from build123d import *

# Parameters (mm, degrees)
F0_R      = 42.199156
F1_DEPTH  = 50.8
F2_R      = 26.140573
F3_DEPTH  = 25.4
F4_R      = 17.712335
F5_DEPTH  = 25.4
F6_R      = 23.120753
F1_FACE_R = 42.199156
F7_DEPTH  = 50.8
F8_R      = 26.373647
F9_DEPTH  = 76.2
F10_R     = 19.05
F11_DEPTH = 254
F12_R     = 5.08


with BuildPart() as f1:
    # F0 (on Front) → F1 (new body)
    with BuildSketch(Plane.XZ):
        Circle(F0_R)
    extrude(amount=F1_DEPTH)

    # F2 (on Front) → F3 (join)
    with BuildSketch(Plane.XZ):
        Circle(F2_R)
    extrude(amount=F3_DEPTH)

    # F4 (on Front) → F5 (join)
    with BuildSketch(Plane.XZ):
        Circle(F4_R)
    extrude(amount=F5_DEPTH)

    # F6 (on Front) + F1_face (on face) → F7 (join)
    with BuildSketch(Plane.XZ):
        Circle(F6_R)
    with BuildSketch(Plane.XZ.offset(50.8)):
        Circle(F1_FACE_R)
    extrude(amount=F7_DEPTH)

    # F8 (on face) → F9 (join)
    with BuildSketch(Plane.XZ.offset(101.6)):
        Circle(F8_R)
    extrude(amount=F9_DEPTH)

    # F10 (on face) → F11 (cut)
    with BuildSketch(Plane.XZ.offset(177.8)):
        Circle(F10_R)
    extrude(amount=-F11_DEPTH, mode=Mode.SUBTRACT)

    # F12
    f12_edges = [f1.edges().sort_by_distance(p)[0] for p in [
        (-26.373647, -177.8, 0),
    ]]
    fillet(f12_edges, radius=F12_R)


solid = f1.part
Work out the finished part from the listing and answer in its coordinate system (mm). A direction names the side the tool comes from. Round coordinates to 2 decimals unless told otherwise and drop trailing zeros. Order: outer loops, then holes, each group sorted by start corner. A loop starts at its lowest first (then second) coordinate and runs counter-clockwise, first axis right, second up. Notation, with made-up numbers: M 24,51.25 L 41,51.25 A19 cw 41,74.25 Z; hole C 13.5,14 d4. An arc over 180 degrees is marked long. Put each result on its own line as item: value. Start each with the question number.
Q1. Straight lines are drawn through the part: L1, parallel to Z at x = 0, y = -87; L2, parallel to Z at x = 0, y = -141; L3, parallel to Y at x = 15.5, z = 34. For each, find the intervals that lie inside material, in ascending order. Write a range as [from, to].
Q2. Section A-A, the plane x = 0 is taken. Write down the section's boundary in (y, z).
Q3. Section C-C, the plane y = -38 is taken. Write down the section's boundary in (x, z).
Q4. Flat-ended cylindrical pins translate along their axes: pin 1 (12 mm diameter, centred on x = -25, y = -21, fed in from +Z); pin 2 (5 mm diameter, centred on x = 1, y = -142.5, fed in from +Z); pin 3 (4 mm diameter, centred on x = 11.5, y = -60, fed in from -Z); pin 4 (12 mm diameter, centred on x = 22, z = 15.5, fed in from -Y). Find the tip coordinate at first contact, or state that the pin passes through.
Q5. Section B-B, the plane z = 0 is taken. Write down the section's boundary in (x, y).
Q6. Section D-D, the plane x = 29 is taken. Write down the section's boundary in (y, z), and give its area (3 significant figures).
Q7. For a pull along X with two mould halves and no side action, classify faces 1 (the cylindrical face through (-5.717, -136.662, -25.746)), 2 (the cylindrical face through (-15.12, -90.14, -11.59)), 3 (the flat face through (18, 0, -9)) as pulls with the +X half, pulls with the -X half, needs draft (parallel to the pull), parting line crosses it, or undercut.
Q8. A tool of negligible diameter and unlimited length cuts with its end or side. For faces 4 (the flat face through (-16, -177.8, -11)), 5 (the flat face through (-19.3, -101.6, -18.2)), from which of +Z, -Z, +X, -X, +Y, -Y can it reach the whole face along a straight path? Write none if from no direction.
Findings below:
1. L1: z = [-42.2, -19.05], [19.05, 42.2]
1. L2: z = [-26.37, -19.05], [19.05, 26.37]
1. L3: y = [-101.6, 0]
2. outline: M -177.8,-21.29 A5.08 ccw -172.72,-26.37 L -101.6,-26.37 L -101.6,-42.2 L 0,-42.2 L 0,-19.05 L -177.8,-19.05 Z; M -177.8,19.05 L 0,19.05 L 0,42.2 L -101.6,42.2 L -101.6,26.37 L -172.72,26.37 A5.08 ccw -177.8,21.29 Z
3. outline: C 0,0 d84.4; hole C 0,0 d38.1
4. pin 1: stops at z = 37.68
4. pin 2: stops at z = 26.37
4. pin 3: stops at z = -41.12
4. pin 4: stops at y = -177.8
5. outline: M -42.2,-101.6 L -26.37,-101.6 L -26.37,-172.72 A5.08 ccw -21.29,-177.8 L -19.05,-177.8 L -19.05,0 L -42.2,0 Z; M 19.05,-177.8 L 21.29,-177.8 A5.08 ccw 26.37,-172.72 L 26.37,-101.6 L 42.2,-101.6 L 42.2,0 L 19.05,0 Z
6. outline: M -101.6,-30.66 L 0,-30.66 L 0,30.66 L -101.6,30.66 Z
6. area: 6,230 mm^2
7. face 1: parting line crosses it
7. face 2: undercut
7. face 3: needs draft
8. face 4: +Z, -Z, +X, -X, -Y
8. face 5: -Y
